Could you check a few things on this model? Use its own coordinates, in mm. A direction names the side the tool comes from. Coordinates: 2 decimals unless noted, no trailing zeros. Order: outer loops, then holes, each group sorted by start corner. A loop starts at its lowest first (then second) coordinate and runs counter-clockwise, first axis right, second up. Notation, with made-up numbers: (64, 68.5) -> (122, 68.5) arc R21 cw to (122, 83.5) -> close; hole circle Ø5 at (48.25, 31.25). An arc over 180 degrees is marked (long way). Return JSON: item names as keys, results as strings. Group by question number.
from build123d import *

# Parameters (mm, degrees)
MAINGEAR_DEPTH                     = 10
CONG_1_R                           = 0.45
R_P_TITION_CIRCULAIRE1_COUNT       = 4
R_P_TITION_CIRCULAIRE1_ANGLE       = 90
CONG_1_OF_R_P_TITION_CIRCULAIRE1_R = 0.45
ESQUISSE5_R                        = 7.125
MAINBASECIRCLE_DEPTH               = 10
REMOVEGEARTOP_DEPTH                = 10
ESQUISSE9_R                        = 7.125
ESQUISSE9_R_2                      = 3.1
GEARBOTTOMFIX_DEPTH                = 12
ESQUISSE3_R                        = 3.1
GEARHOLE_DEPTH                     = 23
MEPLATHOLE_DEPTH                   = 15


with BuildPart() as part:
    # Esquisse1 → MainGear (new body)
    with BuildSketch(Plane.XY):
        with BuildLine():
            Line((0, 0), (6.882221512, 1.844085696))
            ThreePointArc((6.882221512, 1.844085696), (6.988095123, 1.390018544), (7.064044637, 0.92999912))
            Line((7.064044637, 0.92999912), (8.384880781, 1.103890497))
            ThreePointArc((8.384880781, 1.103890497), (9.465680859, 1.068283463), (10.477518694, 0.686732857))
            ThreePointArc((10.477518694, 0.686732857), (10.5, 0), (10.477518694, -0.686732857))
            ThreePointArc((10.477518694, -0.686732857), (9.465680859, -1.068283463), (8.384880781, -1.103890497))
            Line((8.384880781, -1.103890497), (7.064044637, -0.92999912))
            ThreePointArc((7.064044637, -0.92999912), (6.988095123, -1.390018544), (6.882221512, -1.844085696))
            Line((6.882221512, -1.844085696), (0, 0))
        make_face()
    maingear = extrude(amount=MAINGEAR_DEPTH)

    # Cong_1
    cong_1_edges = [part.edges().sort_by_distance(p)[0] for p in [
        (7.064044637, 0.92999912, 5),
        (7.064044637, -0.92999912, 5),
    ]]
    fillet(cong_1_edges, radius=CONG_1_R)

    # R_p_tition circulaire1: MainGear ×4 about axis
    r_p_tition_circulaire1_axis = Axis((0, 0, 0), (0, 0, -1))
    for i in range(1, R_P_TITION_CIRCULAIRE1_COUNT):
        add(maingear.rotate(r_p_tition_circulaire1_axis, i * R_P_TITION_CIRCULAIRE1_ANGLE / (R_P_TITION_CIRCULAIRE1_COUNT - 1)))

    # Cong_1 of R_p_tition circulaire1
    cong_1_of_r_p_tition_circulaire1_edges = [part.edges().sort_by_distance(p)[0] for p in [
        (6.582641669, -2.726619456, 5),
        (5.65264255, -4.337425182, 5),
        (4.337425182, -5.65264255, 5),
        (2.726619456, -6.582641669, 5),
        (0.92999912, -7.064044637, 5),
        (-0.92999912, -7.064044637, 5),
    ]]
    fillet(cong_1_of_r_p_tition_circulaire1_edges, radius=CONG_1_OF_R_P_TITION_CIRCULAIRE1_R)

    # Esquisse9 → GearBottomFix (add)
    with BuildSketch(Plane.XY.offset(10)):
        Circle(ESQUISSE9_R)
        Circle(ESQUISSE9_R_2, mode=Mode.SUBTRACT)
    extrude(amount=GEARBOTTOMFIX_DEPTH)


with BuildPart() as body_2:
    # Esquisse5 → MainBaseCircle (new body, through all)
    with BuildSketch(Plane.XY.offset(10)):
        Circle(ESQUISSE5_R)
    extrude(amount=-MAINBASECIRCLE_DEPTH)

    # Esquisse7 → RemoveGearTop (cut)
    with BuildSketch(Plane.XY.offset(10)):
        with BuildLine():
            Line((-6.868119582, -1.895932068), (-1.792134456, 6.895932068))
            ThreePointArc((-1.792134456, 6.895932068), (-6.170431002, 3.5625), (-6.868119582, -1.895932068))
        make_face()
    extrude(amount=-REMOVEGEARTOP_DEPTH, mode=Mode.SUBTRACT)


with BuildPart() as gearhole_tool:
    # Esquisse3 → GearHole (new body, through all)
    with BuildSketch(Plane.XY):
        Circle(ESQUISSE3_R)
    extrude(amount=GEARHOLE_DEPTH)


with BuildPart() as part_1:
    add(part.part)

    # GearHole: cut by gearhole_tool
    add(gearhole_tool.part, mode=Mode.SUBTRACT)



with BuildPart() as body_2_1:
    add(body_2.part)

    # GearHole: cut by gearhole_tool
    add(gearhole_tool.part, mode=Mode.SUBTRACT)


with BuildPart() as part_2:
    add(part_1.part)

    add(body_2_1.part)  # MeplatHole merges body 2
    # Esquisse10 → MeplatHole (add)
    with BuildSketch(Plane(origin=(0, 0, 0), x_dir=(-1, 0, 0), z_dir=(0, 0, -1))):
        with BuildLine():
            Line((-1.24854837, -2.837450787), (-3.081578648, 0.337450787))
            ThreePointArc((-3.081578648, 0.337450787), (-2.684678752, -1.55), (-1.24854837, -2.837450787))
        make_face()
    extrude(amount=-MEPLATHOLE_DEPTH)


solid = part_2.part
Q1. I want a section at C-C on z = 13.25. Please give me the cut outline in (x, y) (3 decimals).
Q2. On a 3-axis mill with a long thin cutter (end or side, diameter ignored), from which of +Z, -Z, +X, -X, +Y, -Y can I reach the whole of each face in a straight line? I mean faces 1 (the cylindrical face through (1.07, -9.45, 4.93)), 2 (the cylindrical face through (5.653, -7.649, 4.93)), 3 (the flat face through (-1.046, -7.947, 4.93)), 4 (the flat face through (-5, 3, 10)). Say none if no direction works.
Q3. I want a section at D-D on y = -9. Please give me the cut outline in (x, z).
Q4. I'm going to push flat-ended pins straight in: pin 1 Ø2 at (x, y) = (9, -0.5) entering from +Z; pin 2 Ø1 at (x, z) = (-1, 12) entering from -Y; pin 3 Ø4 at (x, z) = (-5, 17) entering from +Y. Where does each tip first touch, or does it pass through?
Q5. I want a section at A-A on x = 0. Please give me the cut outline in (y, z) (3 decimals).
Q6. We'd pull the mould along Y, two halves only. Please class faces 5 (the flat face through (2.4, -1.4, 15)), 6 (the cylindrical face through (0, -10.5, 4.9)), 7 (the cylindrical face through (8.72, -3.8, 4.93)), 8 (the flat face through (0, -9, 10)): pulls with the +Y half, pulls with the -Y half, needs draft (parallel to the pull), parting line crosses it, or undercut.
Q7. I need wall thicknesses on line 1 along X through (y, z) = (0, 12.25) (3 decimals); line 2 along Y through (x, z) = (0, 7.75) (3 decimals); line 3 along Y through (x, z) = (0, 13.75) (3 decimals). Which ranges of each line are inside material? Lowest first, please. Write a range as from..to.
Response values:
{
 "1": {"outline": "circle Ø14.25 at (0, 0); hole (1.249, -2.837) -> (3.082, 0.337) arc R3.1 ccw (long way) to start"},
 "2": {"face 1": "+Z, -Z", "face 2": "+Z, -Z, +X", "face 3": "+Z, -Z, -X", "face 4": "-Z, -X, +Y"},
 "3": {"outline": "(-1.13, 0) -> (1.13, 0) -> (1.13, 10) -> (-1.13, 10) -> close; (4.07, 0) -> (5.41, 0) -> (5.41, 10) -> (4.07, 10) -> close"},
 "4": {"pin 1": "stops at z = 10", "pin 2": "stops at y = -7.11", "pin 3": "stops at y = 6.46"},
 "5": {"outline": "(-10.5, 0) -> (-3.1, 0) -> (-3.1, 22) -> (-7.125, 22) -> (-7.125, 10) -> (-10.5, 10) -> close; (3.1, 0) -> (7.125, 0) -> (7.125, 22) -> (3.1, 22) -> close"},
 "6": {"face 5": "undercut", "face 6": "pulls with the -Y half", "face 7": "undercut", "face 8": "needs draft"},
 "7": {"line 1": "x = -7.125..-3.1, 2.887..7.125", "line 2": "y = -10.5..-3.1, 3.1..7.125", "line 3": "y = -7.125..-3.1, 3.1..7.125"}
}
